Here's how the part is built. I have some questions about the finished solid (model axes, mm). A direction names the side the tool comes from. Give positions to 0.01 mm unless a question says otherwise; leave off trailing zeros. Order: outer loops, then holes, each group sorted by start corner. A loop starts at its lowest first (then second) coordinate and runs counter-clockwise, first axis right, second up. Notation, with made-up numbers: M -32.5,-1.5 L -0.5,-1.5 A12 ccw -0.5,11.5 Z; hole C -17.75,11 d6. An arc over 180 degrees is marked long. Use one line per item in the form item = value.
from build123d import *

# Parameters (mm, degrees)
SKETCH1_R           = 49.5
BOSS_EXTRUDE1_DEPTH = 2
BOSS_EXTRUDE1_TAPER = 1
SKETCH2_R           = 4
HOLDER_DEPTH        = 15
HOLDERCUT_DEPTH     = 5
FILLET1_R           = 2
SKETCH6_R           = 7.15
CAMCUT_DEPTH        = 11
CAMCUT_DRAFT        = -1
CUT_EXTRUDE1_DEPTH  = 10
SKETCH8_R           = 49.5
BOSS_EXTRUDE2_DEPTH = 8.5
BOSS_EXTRUDE2_TAPER = 1
SKETCH9_R           = 47.851631948
SKETCH9_R_2         = 4
CUT_EXTRUDE5_DEPTH  = 5
SKETCH10_R          = 7.15
CUT_EXTRUDE6_DEPTH  = 10


with BuildPart() as part:
    # Sketch1 → Boss-Extrude1 (new body)
    with BuildSketch(Plane.XY):
        Circle(SKETCH1_R)
    extrude(amount=BOSS_EXTRUDE1_DEPTH, taper=BOSS_EXTRUDE1_TAPER)

    # Sketch2 → Holder (add)
    with BuildSketch(Plane.XY.offset(2)):
        with Locations((0.029161528, 0.006821447)):
            Circle(SKETCH2_R)
    extrude(amount=-HOLDER_DEPTH)

    # Sketch5 → HolderCut (cut)
    with BuildSketch(Plane(origin=(0, 0, -13), x_dir=(-1, 0, 0), z_dir=(0, 0, -1))):
        with BuildLine():
            Line((-1.576483824, 2.191962306), (-1.576483824, -2.191962306))
            ThreePointArc((-1.576483824, -2.191962306), (2.7, 0), (-1.576483824, 2.191962306))
        make_face()
    extrude(amount=-HOLDERCUT_DEPTH, mode=Mode.SUBTRACT)

    # Fillet1
    fillet1_edges = [part.edges().sort_by_distance(p)[0] for p in [
        (-49.46508987, 0, 2),
    ]]
    fillet(fillet1_edges, radius=FILLET1_R)


with BuildPart() as camcut_tool:
    # Sketch6 → CamCut (with draft: the straight prism first)
    with BuildSketch(Plane.XY.offset(2)):
        with Locations((2.075653978, 29.594808325)):
            Circle(SKETCH6_R)
    extrude(amount=-CAMCUT_DEPTH)
    # CamCut: the draft: its side faces are tilted about the plane it starts from
    camcut_sides = [camcut_tool.faces().sort_by_distance(p)[0] for p in [
        (-5.074346022, 29.594808325, -3.5),
    ]]
    draft(camcut_sides, Plane.XY.offset(2), CAMCUT_DRAFT)


with BuildPart() as part_1:
    add(part.part)

    # CamCut: cut by camcut_tool
    add(camcut_tool.part, mode=Mode.SUBTRACT)

    # Sketch7 → Cut-Extrude1 (cut)
    with BuildSketch(Plane(origin=(0, 0, -13), x_dir=(-1, 0, 0), z_dir=(0, 0, -1))):
        with BuildLine():
            Line((-1.676483824, 2.242632825), (-1.676483824, -2.242632825))
            ThreePointArc((-1.676483824, -2.242632825), (2.8, 0), (-1.676483824, 2.242632825))
        make_face()
    extrude(amount=-CUT_EXTRUDE1_DEPTH, mode=Mode.SUBTRACT)

    # Sketch8 → Boss-Extrude2 (add)
    with BuildSketch(Plane(origin=(0, 0, 0), x_dir=(-1, 0, 0), z_dir=(0, 0, -1))):
        Circle(SKETCH8_R)
    extrude(amount=BOSS_EXTRUDE2_DEPTH, taper=BOSS_EXTRUDE2_TAPER)

    # Sketch9 → Cut-Extrude5 (cut)
    with BuildSketch(Plane(origin=(0, 0, -8.5), x_dir=(-1, 0, 0), z_dir=(0, 0, -1))):
        Circle(SKETCH9_R)
        Circle(SKETCH9_R_2, mode=Mode.SUBTRACT)
    extrude(amount=-CUT_EXTRUDE5_DEPTH, mode=Mode.SUBTRACT)

    # Sketch10 → Cut-Extrude6 (cut)
    with BuildSketch(Plane.XY.offset(2)):
        with Locations((2.075653978, 29.594808325)):
            Circle(SKETCH10_R)
    extrude(amount=-CUT_EXTRUDE6_DEPTH, mode=Mode.SUBTRACT)


solid = part_1.part
Q1. I want a section at B-B on z = -11.25. Write out the boundary of the cut face in (x, y), then the cut area to 3 significant figures.
Found:
outline = C 0.03,0.01 d8; hole M 1.68,-2.24 L 1.68,2.24 A2.8 ccw long Z
area = 29.2 mm²
Q2. I'm going to push flat-ended pins straight in: pin 1 Ø6 at (x, z) = (22.5, -10.5) entering from -Y; pin 2 Ø1.5 at (y, z) = (30, -4.5) entering from +X; pin 3 Ø2 at (x, y) = (-0.5, -0.5) entering from -Z; pin 4 Ø11.5 at (x, y) = (2.08, 29.59) entering from -Z. Where does each tip first touch, or does it pass through?
Found:
pin_1 = -45
pin_2 = 39.84
pin_3 = -8.5
pin_4 = through
Q3. Thinking about a two-plate mould opening in X: for faces 3 (the face through (2, 0, -13)), 4 (the face through (1.676, 0, -11)), 5 (the face through (3.844, 1.208, -10.718)), which applies, +X half, -X half, draft (parallel to the pull), parting line (faces both ways), or undercut?
Found:
face_3 = draft
face_4 = undercut
face_5 = parting line
Q4. I need wall thicknesses on L1, parallel to Y at x = 0, z = -9.65; L2, parallel to Y at x = 0, z = -6.3; L3, parallel to X at y = 3.5, z = -2. Which ranges of each line are inside material? Lowest first, please.
Found:
L1 = -3.99 to -2.8, 2.8 to 4.01
L2 = -49.39 to -47.85, -4 to 4, 47.85 to 49.39
L3 = -49.34 to 49.34
Q5. On a 3-axis mill with a long thin cutter (end or side, diameter ignored), from which of +Z, -Z, +X, -X, +Y, -Y can I reach the whole of each face in a straight line? I mean faces 1 (the face through (-2.8, -0.1, -10.8)), 2 (the face through (1.145, 36.684, -0.712)). Say none if no direction works.
Found:
face_1 = -Z
face_2 = +Z, -Z
